Here's how the part is built. I have some questions about the finished solid (model axes, mm). Round coordinates to 2 decimals unless told otherwise and drop trailing zeros. Order: outer loops, then holes, each group sorted by start corner. A loop starts at its lowest first (then second) coordinate and runs counter-clockwise, first axis right, second up.
```python
from build123d import *

# Parameters (mm, degrees)
SKETCH1_W           = 200
SKETCH1_H           = 30
BOSS_EXTRUDE1_DEPTH = 3.175
FILLET1_R           = 5
SKETCH2_R           = 2.5
CUT_EXTRUDE1_DEPTH  = 186.634265762
SKETCH3_R           = 1.625
CUT_EXTRUDE3_DEPTH  = 186.634265762
SKETCH4_R           = 1.75
CUT_EXTRUDE4_DEPTH  = 10
SKETCH5_R           = 2.125
CUT_EXTRUDE5_DEPTH  = 186.634265762


with BuildPart() as part:
    # Sketch1 → Boss-Extrude1 (new body)
    with BuildSketch(Plane(origin=(0, 0, 0), x_dir=(1, 0, 0), z_dir=(0, 1, 0))):
        with Locations((85, 0)):
            Rectangle(SKETCH1_W, SKETCH1_H)
    extrude(amount=BOSS_EXTRUDE1_DEPTH)

    # Fillet1
    fillet1_edges = [part.edges().sort_by_distance(p)[0] for p in [
        (-15, 1.5875, -15),
        (185, 1.5875, -15),
        (185, 1.5875, 15),
        (-15, 1.5875, 15),
    ]]
    fillet(fillet1_edges, radius=FILLET1_R)

    # Sketch2 → Cut-Extrude1 (cut, through all)
    with BuildSketch(Plane(origin=(0, 3.175, 0), x_dir=(1, 0, 0), z_dir=(0, 1, 0))):
        with Locations(Location((0, 0, 0), (0, 0, 270))):
            Circle(SKETCH2_R)
    extrude(amount=-CUT_EXTRUDE1_DEPTH, mode=Mode.SUBTRACT)

    # Sketch3 → Cut-Extrude3 (cut, through all)
    with BuildSketch(Plane(origin=(0, 3.175, 0), x_dir=(1, 0, 0), z_dir=(0, 1, 0))):
        with Locations(Location((7.5, 0, 0), (0, 0, 270))):
            Circle(SKETCH3_R)
        with Locations(Location((0, -7.5, 0), (0, 0, 270))):
            Circle(SKETCH3_R)
        with Locations(Location((-7.5, 0, 0), (0, 0, 270))):
            Circle(SKETCH3_R)
        with Locations(Location((0, 7.5, 0), (0, 0, 270))):
            Circle(SKETCH3_R)
    extrude(amount=-CUT_EXTRUDE3_DEPTH, mode=Mode.SUBTRACT)

    # Sketch4 → Cut-Extrude4 (cut)
    with BuildSketch(Plane(origin=(0, 3.175, 0), x_dir=(1, 0, 0), z_dir=(0, 1, 0))):
        with Locations(Location((60, -10, 0), (0, 0, 270))):
            Circle(SKETCH4_R)
        with Locations(Location((110, -10, 0), (0, 0, 270))):
            Circle(SKETCH4_R)
        with Locations(Location((110, 10, 0), (0, 0, 270))):
            Circle(SKETCH4_R)
        with Locations(Location((60, 10, 0), (0, 0, 270))):
            Circle(SKETCH4_R)
    extrude(amount=-CUT_EXTRUDE4_DEPTH, mode=Mode.SUBTRACT)

    # Sketch5 → Cut-Extrude5 (cut, through all)
    with BuildSketch(Plane(origin=(0, 3.175, 0), x_dir=(1, 0, 0), z_dir=(0, 1, 0))):
        with Locations(Location((166, 8, 0), (0, 0, 270))):
            Circle(SKETCH5_R)
        with Locations(Location((178, 8, 0), (0, 0, 90))):
            Circle(SKETCH5_R)
        with Locations(Location((178, -8, 0), (0, 0, 270))):
            Circle(SKETCH5_R)
        with Locations(Location((166, -8, 0), (0, 0, 90))):
            Circle(SKETCH5_R)
    extrude(amount=-CUT_EXTRUDE5_DEPTH, mode=Mode.SUBTRACT)


solid = part.part
```
1) If we section it at A-A (z = 0): Write out the boundary of the cut face in (x, y) (3 decimals), plus the area to 3 significant figures.
2) We'd pull the mould along X, two halves only. Please class faces 1 (the cylindrical face through (180.107, 1.61, 7.723)), 2 (the cylindrical face through (184, 2, -13)), 3 (the flat face through (84, 2, -15)), 4 (the cylindrical face through (168.107, 1.61, -8.277)): +X half, -X half, draft (parallel to the pull), parting line (faces both ways), or undercut.
3) If we section it at C-C (y = 0.75): Give the number of separate pieces and of enclosed holes in the cut face, plus the area to 3 significant figures.
4) If we section it at B-B (x = -7.5): Write out the boundary of the cut face in (y, z) (3 decimals).
5) I need wall thicknesses on line 1 (X direction, y = 1.8, z = 0) (3 decimals); line 2 (Z direction, x = 110, y = 2.45); line 3 (X direction, y = 1.2, z = -8) (3 decimals). Which ranges of each line are inside material? Lowest first, please.
6) If we section it at D-D (x = 178): Write out the boundary of the cut face in (y, z) (3 decimals).
7) I'm going to push a flat-ended pin straight in: pin 1 (4.5 mm diameter, centred on x = 0, z = 0, fed in from +Y). Where does the tip first touch, or does it pass through?
Solutions:
1. outline: (-15, 0) - (-9.125, 0) - (-9.125, 3.175) - (-15, 3.175) - close; (-5.875, 0) - (-2.5, 0) - (-2.5, 3.175) - (-5.875, 3.175) - close; (2.5, 0) - (5.875, 0) - (5.875, 3.175) - (2.5, 3.175) - close; (9.125, 0) - (185, 0) - (185, 3.175) - (9.125, 3.175) - close
1. area: 598 mm2
2. face 1: undercut
2. face 2: +X half
2. face 3: draft
2. face 4: undercut
3. separate pieces: 1
3. enclosed holes: 13
3. area: 5,830 mm2
4. outline: (0, -15) - (3.175, -15) - (3.175, -1.625) - (0, -1.625) - close; (0, 1.625) - (3.175, 1.625) - (3.175, 15) - (0, 15) - close
5. line 1: x = -15 to -9.125, -5.875 to -2.5, 2.5 to 5.875, 9.125 to 185
5. line 2: z = -15 to -11.75, -8.25 to 8.25, 11.75 to 15
5. line 3: x = -15 to -1.546, 1.546 to 163.875, 168.125 to 175.875, 180.125 to 185
6. outline: (0, -15) - (3.175, -15) - (3.175, -10.125) - (0, -10.125) - close; (0, -5.875) - (3.175, -5.875) - (3.175, 5.875) - (0, 5.875) - close; (0, 10.125) - (3.175, 10.125) - (3.175, 15) - (0, 15) - close
7. pin 1: passes through
